from build123d import *

# Parameters (mm, degrees)
CROQUIS1_W              = 60
CROQUIS1_H              = 150
CROQUIS1_R              = 1.5
CROQUIS1_R_2            = 2.5
CROQUIS1_R_3            = 4.25
CROQUIS1_R_4            = 7.5
SALIENTE_EXTRUIR1_DEPTH = 6
CHAFL_N1_SIZE           = 0.5


with BuildPart() as part:
    # Croquis1 → Saliente-Extruir1 (new body)
    with BuildSketch(Plane(origin=(0, 0, 0), x_dir=(1, 0, 0), z_dir=(0, 1, 0))):
        with Locations((-9.728313692, -1.041413592)):
            Rectangle(CROQUIS1_W, CROQUIS1_H)
        with Locations(Location((-32.228313692, 28.958586408, 0), (0, 0, 270))):
            Circle(CROQUIS1_R, mode=Mode.SUBTRACT)
        with Locations(Location((-32.228313692, -31.041413592, 0), (0, 0, 270))):
            Circle(CROQUIS1_R, mode=Mode.SUBTRACT)
        with Locations(Location((5.271686308, 17.208586408, 0), (0, 0, 270))):
            Circle(CROQUIS1_R_2, mode=Mode.SUBTRACT)
        with Locations(Location((5.271686308, -19.291413592, 0), (0, 0, 270))):
            Circle(CROQUIS1_R_2, mode=Mode.SUBTRACT)
        with Locations(Location((-32.228313692, 58.958586408, 0), (0, 0, 270))):
            Circle(CROQUIS1_R, mode=Mode.SUBTRACT)
        with Locations(Location((-32.228313692, -61.041413592, 0), (0, 0, 270))):
            Circle(CROQUIS1_R, mode=Mode.SUBTRACT)
        with Locations(Location((5.271686308, -1.041413592, 0), (0, 0, 270))):
            Circle(CROQUIS1_R_3, mode=Mode.SUBTRACT)
        with Locations(Location((-32.228313692, -1.041413592, 0), (0, 0, 270))):
            Circle(CROQUIS1_R, mode=Mode.SUBTRACT)
        with Locations(Location((5.271686308, -51.041413592, 0), (0, 0, 270))):
            Circle(CROQUIS1_R_4, mode=Mode.SUBTRACT)
        with Locations(Location((5.271686308, 48.958586408, 0), (0, 0, 270))):
            Circle(CROQUIS1_R_4, mode=Mode.SUBTRACT)
        with Locations(Location((5.271686308, 66.958586408, 0), (0, 0, 270))):
            Circle(CROQUIS1_R_2, mode=Mode.SUBTRACT)
        with Locations(Location((5.271686308, 30.958586408, 0), (0, 0, 270))):
            Circle(CROQUIS1_R_2, mode=Mode.SUBTRACT)
        with Locations(Location((5.271686308, -33.041413592, 0), (0, 0, 270))):
            Circle(CROQUIS1_R_2, mode=Mode.SUBTRACT)
        with Locations(Location((5.271686308, -69.041413592, 0), (0, 0, 270))):
            Circle(CROQUIS1_R_2, mode=Mode.SUBTRACT)
    extrude(amount=SALIENTE_EXTRUIR1_DEPTH)

    # Chafl_n1
    chafl_n1_edges = [part.edges().sort_by_distance(p)[0] for p in [
        (20.271686308, 6, 1.041413592),
        (-32.228313692, 0, -30.458586408),
        (-32.228313692, 6, -30.458586408),
        (-9.728313692, 6, -73.958586408),
        (-32.228313692, 0, 29.541413592),
        (-32.228313692, 6, 29.541413592),
        (5.271686308, 0, -19.708586408),
        (5.271686308, 6, -19.708586408),
        (5.271686308, 0, 16.791413592),
        (5.271686308, 6, 16.791413592),
        (-32.228313692, 0, -60.458586408),
        (-32.228313692, 6, -60.458586408),
        (-32.228313692, 0, 59.541413592),
        (-32.228313692, 6, 59.541413592),
        (5.271686308, 0, -3.208586408),
        (5.271686308, 6, -3.208586408),
        (-32.228313692, 0, -0.458586408),
        (-32.228313692, 6, -0.458586408),
        (-39.728313692, 6, 1.041413592),
        (5.271686308, 0, 43.541413592),
        (5.271686308, 6, 43.541413592),
        (-9.728313692, 0, -73.958586408),
        (5.271686308, 0, -56.458586408),
        (5.271686308, 6, -56.458586408),
        (20.271686308, 0, 1.041413592),
        (5.271686308, 0, -69.458586408),
        (5.271686308, 6, -69.458586408),
        (-9.728313692, 0, 76.041413592),
        (5.271686308, 0, -33.458586408),
        (5.271686308, 6, -33.458586408),
        (-39.728313692, 0, 1.041413592),
        (5.271686308, 0, 30.541413592),
        (5.271686308, 6, 30.541413592),
        (5.271686308, 0, 66.541413592),
        (5.271686308, 6, 66.541413592),
        (-9.728313692, 6, 76.041413592),
        (-39.728313692, 3, -73.958586408),
        (20.271686308, 3, -73.958586408),
        (20.271686308, 3, 76.041413592),
        (-39.728313692, 3, 76.041413592),
    ]]
    chamfer(chafl_n1_edges, length=CHAFL_N1_SIZE)


solid = part.part
Read the model definition and answer for the solid it produces. Units are mm, in the model's axes. Give positions to 0.01 mm unless a question says otherwise; leave off trailing zeros. Answer as a JSON object with one key per item and string values. Group by question number.
1) Consider L1, parallel to Z at x = -31, y = 3.5; L2, parallel to X at y = 2.25, z = -30; L3, parallel to X at y = 5.5, z = 60. Determine where each line is inside the solid, lowest interval first. Write a range as from..to.
2) Find section A-A (y = 2.75). Count the separate pieces of the cut face and the enclosed holes in it, and give its area (3 significant figures).
3) This flat-tipped pin is pushed along its axis until it touches: P1, Ø3.5, axis at x = -32.23, z = -28.96, coming from the +Y side. Where does it stop, or does it pass through?
Values follow:
{
 "1": {"L1": "z = -73.96..-59.82, -58.1..-29.82, -28.1..0.18, 1.9..30.18, 31.9..60.18, 61.9..76.04", "L2": "x = -39.73..-33.31, -31.15..2.96, 7.58..20.27", "L3": "x = -39.73..-33.31, -31.15..20.27"},
 "2": {"separate pieces": "1", "enclosed holes": "14", "area": "8,440 mm2"},
 "3": {"P1": "stops at y = 5.75"}
}
